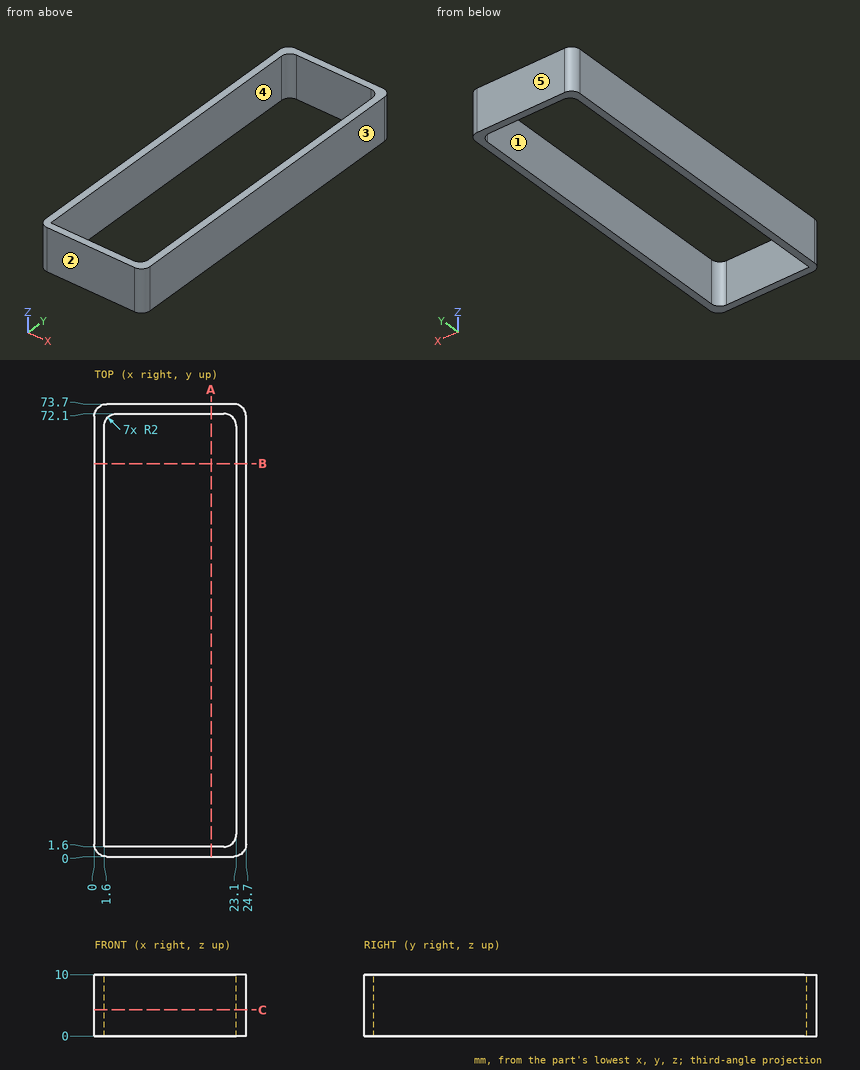
Geometry check sheet. Reference: drawing and pictorial views, mm from the part's lowest x, y, z. A direction names the side the tool comes from. Give positions to 0.01 mm unless a question says otherwise; leave off trailing zeros. Order: outer loops, then holes, each group sorted by start corner. A loop starts at its lowest first (then second) coordinate and runs counter-clockwise, first axis right, second up. Notation, with made-up numbers: (-12.5, -35.75) - (19.5, -35.75) arc R17 ccw to (19.5, -7.75) - close; hole circle Ø2 at (68.25, 19.5). An arc over 180 degrees is marked (long way). Answer as CSV lines item,"result". Start each with the question number.
Item 1: Section check A-A, the plane x = 19. Record the boundary of the cut face in (y, z).
Item 2: Mould release check, pull along Y, two halves, no side actions. Record for the marked faces 1, 2 and 3: released by +Y, released by -Y, zero draft, split by the parting line, or undercut.
Item 3: Section check B-B, the plane y = 64. Record the boundary of the cut face in (x, z).
Item 4: Section check C-C, the plane z = 4.25. Record the boundary of the cut face in (x, y).
Item 5: Access from +Z, -Z, +X, -X, +Y, -Y to the whole of each face (thin tool, end or side, straight path). Record for the marked faces 4 and 5.
Item 6: Material ranges on L1, parallel to X at y = 37, z = 7.25; L2, parallel to Y at x = 13, z = 1; L3, parallel to Y at x = 1.5, z = 4.25, recorded low to high.
Filled in:
1,outline,"(0, 0) - (1.6, 0) - (1.6, 10) - (0, 10) - close; (72.1, 0) - (73.7, 0) - (73.7, 10) - (72.1, 10) - close"
2,face 1,"undercut"
2,face 2,"released by -Y"
2,face 3,"zero draft"
3,outline,"(0, 0) - (1.6, 0) - (1.6, 10) - (0, 10) - close; (23.1, 0) - (24.7, 0) - (24.7, 10) - (23.1, 10) - close"
4,outline,"(0, 2) arc R2 ccw to (2, 0) - (22.7, 0) arc R2 ccw to (24.7, 2) - (24.7, 71.7) arc R2 ccw to (22.7, 73.7) - (2, 73.7) arc R2 ccw to (0, 71.7) - close; hole (1.6, 1.6) - (21.1, 1.6) arc R2 ccw to (23.1, 3.6) - (23.1, 70.1) arc R2 ccw to (21.1, 72.1) - (3.6, 72.1) arc R2 ccw to (1.6, 70.1) - close"
5,face 4,"+Z, -Z"
5,face 5,"+Z, -Z, +X, -X, +Y"
6,L1,"0 to 1.6, 23.1 to 24.7"
6,L2,"0 to 1.6, 72.1 to 73.7"
6,L3,"0.06 to 73.64"
